Can you work these out from the model? Positions are in its coordinate system, mm. A direction names the side the tool comes from. Coordinates: 2 decimals unless noted, no trailing zeros. Write each loop counter-clockwise with the first axis right and the second up, starting at its lowest first coordinate (ties: lowest second). Pieces come first, ordered by that corner, then holes. Notation, with made-up numbers: (-31.5, 82) -> (23.5, 82) arc R14 ccw to (23.5, 108) -> close; hole circle Ø11 at (-7.5, 47). An arc over 180 degrees is marked (long way). Answer as CSV lines item,"result". Start each with the question number.
```python
from build123d import *

# Parameters (mm, degrees)
CUT_EXTRUDE1_DEPTH = 3
FILLET1_R          = 0.25


with BuildPart() as part:
    # Sketch2 → Revolve1 (revolve)
    with BuildSketch(Plane.XY, mode=Mode.PRIVATE) as revolve1_sk:
        Polygon((0, 4), (3.5, 4), (3.5, 0), (2, 0), (2, -10), (0, -10), align=None)
    revolve(revolve1_sk.sketch.rotate(Axis((0, 21.322324325, 0), (0, -1, 0)), 180), axis=Axis((0, 21.322324325, 0), (0, -1, 0)))

    # Sketch3 → Cut-Extrude1 (cut)
    with BuildSketch(Plane(origin=(0, 4, 0), x_dir=(1, 0, 0), z_dir=(0, 1, 0))):
        Polygon((2.020725942, 0), (1.010362971, 1.75), (-1.010362971, 1.75), (-2.020725942, 0), (-1.010362971, -1.75), (1.010362971, -1.75), align=None)
    extrude(amount=-CUT_EXTRUDE1_DEPTH, mode=Mode.SUBTRACT)

    # Fillet1
    fillet1_edges = [part.edges().sort_by_distance(p)[0] for p in [
        (1.515544457, 4, 0.875),
        (1.515544457, 4, -0.875),
        (0, 4, -1.75),
        (-1.515544457, 4, -0.875),
        (-1.515544457, 4, 0.875),
        (0, 4, 1.75),
        (2, 0, 0),
        (3.5, 0, 0),
        (3.5, 4, 0),
    ]]
    fillet(fillet1_edges, radius=FILLET1_R)


solid = part.part
```
Q1. Which directions (+Z, -Z, +X, -X, +Y, -Y) give clear straight access to the entire face, cutting with the end or side of a thin tool? Please do faces 1 (the face through (0, -10, 0)), 2 (the face through (0, -5, 2)), 3 (the face through (-1.5, 2.4, -0.9)).
Q2. I need wall thicknesses on L1, parallel to Y at x = -1, z = 2.5; L2, parallel to Z at x = 0, y = -7; L3, parallel to Y at x = 0.5, z = 1. Which ranges of each line are inside material? Lowest first, please.
Q3. If we mould it in two halves opening along X, with no side actions, what happens to faces 4 (the face through (2, 4, 1)), 5 (the face through (-3.233, 1.976, 1.341)), 6 (the face through (0, 1, 0))? For each: released by +X, released by -X, zero draft, split by the parting line, or undercut.
Q4. Imagine slicing it at B-B (y = 1.5). Write out the boundary of the cut face in (x, z).
Q5. Imagine slicing it at A-A (x = 0). Write out the boundary of the cut face in (y, z).
Q6. Imagine slicing it at C-C (y = -1). Write out the boundary of the cut face in (x, z), then the cut area to 3 significant figures.
Q7. For pin 1 (1.5 mm diameter, centred on x = 0, y = -1.5, fed in from +Z); pin 2 (2 mm diameter, centred on x = 2, y = -8.5, fed in from -Z); pin 3 (2 mm diameter, centred on x = 1, y = -4, fed in from -Z), each with a flat end and sliding along its axis, tell me the tip position at first contact or that it passes through.
Entries:
1,face 1,"+Z, -Z, +X, -X, -Y"
1,face 2,"-Y"
1,face 3,"+Y"
2,L1,"0 to 4"
2,L2,"-2 to 2"
2,L3,"-10 to 1"
3,face 4,"zero draft"
3,face 5,"split by the parting line"
3,face 6,"undercut"
4,outline,"circle Ø7 at (0, 0); hole (-2.02, 0) -> (-1.01, -1.75) -> (1.01, -1.75) -> (2.02, 0) -> (1.01, 1.75) -> (-1.01, 1.75) -> close"
5,outline,"(-10, -2) -> (-0.25, -2) arc R0.25 cw to (0, -2.25) -> (0, -3.25) arc R0.25 ccw to (0.25, -3.5) -> (3.75, -3.5) arc R0.25 ccw to (4, -3.25) -> (4, -2) arc R0.25 ccw to (3.75, -1.75) -> (1, -1.75) -> (1, 1.75) -> (3.75, 1.75) arc R0.25 ccw to (4, 2) -> (4, 3.25) arc R0.25 ccw to (3.75, 3.5) -> (0.25, 3.5) arc R0.25 ccw to (0, 3.25) -> (0, 2.25) arc R0.25 cw to (-0.25, 2) -> (-10, 2) -> close"
6,outline,"circle Ø4 at (0, 0)"
6,area,"12.6 mm2"
7,pin 1,"z = 2"
7,pin 2,"z = -1.73"
7,pin 3,"z = -2"
